```python
from build123d import *

# Parameters (mm, degrees)
SKETCH1_R                 = 12.7
BOSS_EXTRUDE1_DEPTH       = 6.35
SKETCH2_R                 = 9.525
BOSS_EXTRUDE2_DEPTH       = 6.35
SKETCH3_R                 = 3.175
CUT_EXTRUDE1_DEPTH        = 12.7
F_6_32_TAPPED_HOLE1_D     = 2.7051
F_6_32_TAPPED_HOLE1_DEPTH = 9.524
F_6_32_TAPPED_HOLE1_TIP   = 0.81269403


with BuildPart() as part:
    # Sketch1 → Boss-Extrude1 (new body)
    with BuildSketch(Plane.XY):
        Circle(SKETCH1_R)
    extrude(amount=BOSS_EXTRUDE1_DEPTH)

    # Sketch2 → Boss-Extrude2 (add)
    with BuildSketch(Plane.XY.offset(6.35)):
        Circle(SKETCH2_R)
    extrude(amount=BOSS_EXTRUDE2_DEPTH)

    # Sketch3 → Cut-Extrude1 (cut)
    with BuildSketch(Plane.XY.offset(12.7)):
        Circle(SKETCH3_R)
    extrude(amount=-CUT_EXTRUDE1_DEPTH, mode=Mode.SUBTRACT)

    # Sketch4 → Cut-Revolve1 (revolve, cut)
    with BuildSketch(Plane(origin=(0, 0, 0), x_dir=(1, 0, 0), z_dir=(0, 1, 0)), mode=Mode.PRIVATE) as cut_revolve1_sk:
        with BuildLine():
            Line((12.7, 0), (12.7, -6.35))
            ThreePointArc((12.7, -6.35), (9.525, -3.175), (12.7, 0))
        make_face()
    revolve(cut_revolve1_sk.sketch.rotate(Axis((0, 0, -3.575887172), (0, 0, 1)), 180), axis=Axis((0, 0, -3.575887172), (0, 0, 1)), mode=Mode.SUBTRACT)

    # #6-32 Tapped Hole1
    with Locations(Plane(origin=(-9.4e-08, 9.525, 9.584004604), x_dir=(1.0, 9.833e-09, 0), z_dir=(-9.833e-09, 1.0, 0))):
        with Locations((0, 0)):
            Hole(F_6_32_TAPPED_HOLE1_D / 2, depth=F_6_32_TAPPED_HOLE1_DEPTH)
            with Locations((0, 0, -(F_6_32_TAPPED_HOLE1_DEPTH + F_6_32_TAPPED_HOLE1_TIP / 2))):  # 118° drill point
                Cone(0, F_6_32_TAPPED_HOLE1_D / 2, F_6_32_TAPPED_HOLE1_TIP, mode=Mode.SUBTRACT)


solid = part.part
```
Can you work these out from the model? Positions are in its coordinate system, mm. A direction names the side the tool comes from. Round coordinates to 2 decimals unless told otherwise and drop trailing zeros. Loops run counter-clockwise (first coordinate to the right, second up) from the corner with the lowest first, then second, coordinate; pieces in that order, holes last.
Item 1: Suppose I cut it at D-D, the plane z = 10.25. Write out the boundary of the cut face in (x, y) (3 decimals).
Item 2: Will these pins go through, and if not, where does the flat tip stop? pin 1 Ø3 at (y, z) = (1.5, 4) entering from +X; pin 2 Ø3 at (x, z) = (0, 9.58) entering from +Y (3 decimals); pin 3 Ø1 at (y, z) = (3.5, 5.5) entering from +X.
Item 3: Suppose I cut it at C-C, the plane z = 7.5. Write out the boundary of the cut face in (x, y) (3 decimals).
Item 4: Suppose I cut it at A-A, the plane y = 0. Write out the boundary of the cut face in (x, z) (3 decimals), then the cut area to 3 significant figures.
Item 5: Please list where these lines run through material, in increasing order: L1, parallel to Y at x = 0, z = 7 (3 decimals); L2, parallel to Z at x = -0.75, y = 10; L3, parallel to Y at x = -2.5, z = 5.
Item 6: If we mould it in two halves opening along Z, with no side actions, what happens to faces 3 (the flat face through (3, -3, 0)), 4 (the cylindrical face through (0.176, 6.154, 8.243)), 5 (the flat face through (4, 0, 12.7))? For each: +Z half, -Z half, draft (parallel to the pull), parting line (faces both ways), or undercut.
Item 7: Suppose I cut it at B-B, the plane x = 0. Write out the boundary of the cut face in (y, z) (3 decimals).
Item 8: Which directions (+Z, -Z, +X, -X, +Y, -Y) give clear straight access to the entire face, cutting with the end or side of a thin tool? Please do faces 1 (the cylindrical face through (-2.06, -9.3, 9.48)), 2 (the cylindrical face through (-0.69, -3.1, 6.44)).
Reported:
1. outline: (-1.177, 2.949) - (-1.177, 9.452) arc R9.525 ccw (long way) to (1.177, 9.452) - (1.177, 2.949) arc R3.175 cw (long way) to start
2. pin 1: stops at x = 10.44
2. pin 2: stops at y = 9.525
2. pin 3: stops at x = 10.71
3. outline: circle Ø19.05 at (0, 0); hole circle Ø6.35 at (0, 0)
4. outline: (-12.7, 0) - (-3.175, 0) - (-3.175, 12.7) - (-9.525, 12.7) - (-9.525, 6.35) - (-12.7, 6.35) arc R3.175 cw to start; (3.175, 0) - (12.7, 0) arc R3.175 cw to (12.7, 6.35) - (9.525, 6.35) - (9.525, 12.7) - (3.175, 12.7) - close
4. area: 170 mm2
5. L1: y = -9.525 to -3.175, 3.175 to 9.525
5. L2: z = 0 to 1.46, 4.89 to 6.35
5. L3: y = -9.79 to -1.96, 1.96 to 9.79
6. face 3: -Z half
6. face 4: undercut
6. face 5: +Z half
7. outline: (-12.7, 0) - (-3.175, 0) - (-3.175, 12.7) - (-9.525, 12.7) - (-9.525, 6.35) - (-12.7, 6.35) arc R3.175 cw to start; (3.175, 0) - (12.7, 0) arc R3.175 cw to (12.7, 6.35) - (9.525, 6.35) - (9.525, 8.231) - (3.175, 8.231) - close; (3.175, 10.937) - (9.525, 10.937) - (9.525, 12.7) - (3.175, 12.7) - close
8. face 1: +Z
8. face 2: +Z, -Z
